Model file for the job. Use its own axes, mm. A direction names the side the tool comes from. Round coordinates to 2 decimals unless told otherwise and drop trailing zeros. Loops run counter-clockwise (first coordinate to the right, second up) from the corner with the lowest first, then second, coordinate; pieces in that order, holes last.
from build123d import *

# Parameters (mm, degrees)
IZIM1_W                     = 69
IZIM1_H                     = 100
Y_KSEKLIK_EKSTR_ZYON1_DEPTH = 3
IZIM2_W                     = 69
IZIM2_H                     = 100
IZIM2_W_2                   = 63
IZIM2_H_2                   = 94
Y_KSEKLIK_EKSTR_ZYON2_DEPTH = 20
KES_EKSTR_ZYON1_DEPTH       = 70
Y_KSEKLIK_EKSTR_ZYON3_DEPTH = 69
IZIM5_R                     = 3
KES_EKSTR_ZYON2_DEPTH       = 20
Y_KSEKLIK_EKSTR_ZYON4_START = -15
IZIM6_R                     = 3
IZIM6_R_2                   = 2
Y_KSEKLIK_EKSTR_ZYON4_DEPTH = 8


with BuildPart() as part:
    # Çizim1 → Yükseklik-Ekstrüzyon1 (new body)
    with BuildSketch(Plane.XY):
        Rectangle(IZIM1_W, IZIM1_H)
    extrude(amount=Y_KSEKLIK_EKSTR_ZYON1_DEPTH)

    # Çizim2 → Yükseklik-Ekstrüzyon2 (add)
    with BuildSketch(Plane.XY.offset(3)):
        Rectangle(IZIM2_W, IZIM2_H)
        Rectangle(IZIM2_W_2, IZIM2_H_2, mode=Mode.SUBTRACT)
    extrude(amount=Y_KSEKLIK_EKSTR_ZYON2_DEPTH)

    # Çizim3 → Kes-Ekstrüzyon1 (cut, through all)
    with BuildSketch(Plane(origin=(34.5, 0, 0), x_dir=(0, 0, -1), z_dir=(1, 0, 0))):
        Polygon((-23, 50), (0, 25), (0, 50), align=None)
    extrude(amount=-KES_EKSTR_ZYON1_DEPTH, mode=Mode.SUBTRACT)

    # Çizim4 → Yükseklik-Ekstrüzyon3 (add, through all)
    with BuildSketch(Plane(origin=(34.5, 0, 0), x_dir=(0, 0, -1), z_dir=(1, 0, 0))):
        Polygon((-23, 50), (-19.78, 50), (0, 28.5), (0, 25), align=None)
    extrude(amount=-Y_KSEKLIK_EKSTR_ZYON3_DEPTH)

    # Çizim5 → Kes-Ekstrüzyon2 (cut)
    with BuildSketch(Plane(origin=(0, 50, 0), x_dir=(1, 0, 0), z_dir=(0, 1, 0))):
        with Locations((-5, -10.594226135)):
            Circle(IZIM5_R)
        with Locations((5, -10.594226135)):
            Circle(IZIM5_R)
    extrude(amount=-KES_EKSTR_ZYON2_DEPTH, mode=Mode.SUBTRACT)

    # Çizim6 → Yükseklik-Ekstrüzyon4 (add)
    with BuildSketch(Plane(origin=(0, 50, 0), x_dir=(1, 0, 0), z_dir=(0, 1, 0)).offset(Y_KSEKLIK_EKSTR_ZYON4_START)):
        with Locations((-5, -10.594226135)):
            Circle(IZIM6_R)
        with Locations((-5, -10.594226135)):
            Circle(IZIM6_R_2, mode=Mode.SUBTRACT)
        with Locations((5, -10.594226135)):
            Circle(IZIM6_R)
        with Locations((5, -10.594226135)):
            Circle(IZIM6_R_2, mode=Mode.SUBTRACT)
    extrude(amount=Y_KSEKLIK_EKSTR_ZYON4_DEPTH)


solid = part.part
Q1. Probe line 1 (Y direction, x = -6.5, z = 12.5); line 2 (X direction, y = 22.5, z = 19.25); line 3 (Z direction, x = 5, y = 39.25). List the from-to ranges inside material, lowest first.
Q2. Slice it at B-B on x = -17.5. Give the cut face in (y, z), plus the area to 3 significant figures.
Q3. Tool access for faces 4 (the face through (-7, 38.94, 10.51)), 5 (the face through (0, -47, 13)), 6 (the face through (34.5, 1, 11)): list every direction of +Z, -Z, +X, -X, +Y, -Y with a clear straight run to the whole face (end or side of a thin tool).
Q4. Slice it at C-C on y = -37.5. Give the cut face in (x, z), plus the area to 3 significant figures.
Q5. Flat gauge pins, fed straight in: P1, Ø6, axis at x = -9, z = 14.5, coming from the +Y side; P2, Ø3, axis at x = 5, z = 10.59, coming from the +Y side; P3, Ø12, axis at x = -26, y = -3, coming from the +Z side; P4, Ø5, axis at x = -4.5, z = 9, coming from the +Y side. Where does each tip first touch, or does it go through?
Q6. Pull direction Z, two halves, no side cores. Call faces 1 (the face through (3, 38.94, 10.51)), 2 (the face through (0, -10, 0)), 3 (the face through (6, 43, 13)): pulls with the +Z half, pulls with the -Z half, needs draft (parallel to the pull), parting line crosses it, or undercut.
Q7. Slice it at D-D on z = 17. Give the cut face in (x, y), plus the area to 3 significant figures.
Q8. Slice it at A-A on x = 5. Give the cut face in (y, z), plus the area to 3 significant figures.
Reply:
1. line 1: y = -50 to -47, 35 to 43
1. line 2: x = -34.5 to -31.5, 31.5 to 34.5
1. line 3: z = 7.59 to 8.59, 12.59 to 13.59
2. outline: (-50, 0) - (28.5, 0) - (50, 19.78) - (50, 23) - (47, 23) - (47, 20.24) - (28.26, 3) - (-47, 3) - (-47, 23) - (-50, 23) - close
2. area: 369 mm2
3. face 4: +Y
3. face 5: +Z
3. face 6: +Z, -Z, +X, +Y, -Y
4. outline: (-34.5, 0) - (34.5, 0) - (34.5, 23) - (31.5, 23) - (31.5, 3) - (-31.5, 3) - (-31.5, 23) - (-34.5, 23) - close
4. area: 327 mm2
5. P1: stops at y = 47.52
5. P2: stops at y = -47
5. P3: stops at z = 23
5. P4: stops at y = 43
6. face 1: undercut
6. face 2: pulls with the -Z half
6. face 3: needs draft
7. outline: (-34.5, -50) - (34.5, -50) - (34.5, 46.98) - (-34.5, 46.98) - close; hole (-31.5, -47) - (31.5, -47) - (31.5, 43.48) - (-31.5, 43.48) - close
7. area: 991 mm2
8. outline: (-50, 0) - (28.5, 0) - (36.75, 7.59) - (43, 7.59) - (43, 8.59) - (35, 8.59) - (35, 7.59) - (33.25, 7.59) - (28.26, 3) - (-47, 3) - (-47, 23) - (-50, 23) - close; (35, 12.59) - (43, 12.59) - (43, 13.59) - (43.28, 13.59) - (50, 19.78) - (50, 23) - (47, 23) - (47, 20.24) - (39.78, 13.59) - (35, 13.59) - close
8. area: 364 mm2
